The listing builds one solid part. Answer for the finished solid, in the listing's coordinates (mm). Face numbers are marked on the shaded views. A direction names the side the tool comes from. Coordinates: 2 decimals unless noted, no trailing zeros. Write each loop counter-clockwise with the first axis right and the second up, starting at its lowest first coordinate (ties: lowest second). Pieces come first, ordered by that corner, then holes. Notation, with made-up numbers: M 85.5,75.5 L 134.5,75.5 A17 ccw 134.5,108.5 Z; hole C 16,14.25 d3. An arc over 180 degrees is marked long. Answer as CSV lines item,"result".
```python
from build123d import *

# Parameters (mm, degrees)
BOSS_EXTRUDE1_DEPTH      = 30
SKETCH2_W                = 50
SKETCH2_H                = 10
CUT_EXTRUDE1_DEPTH       = 25
SKETCH4_R                = 1.5
BOSS_EXTRUDE2_DEPTH      = 5
SKETCH6_W                = 5.331604391
SKETCH6_H                = 3
SKETCH6_W_2              = 6.668395609
SKETCH6_W_3              = 12
SKETCH6_W_4              = 1.5
SKETCH6_H_2              = 4.5
CUT_EXTRUDE15_DEPTH      = 15
SKETCH7_W                = 30.5
SKETCH7_H                = 3
CUT_EXTRUDE16_DEPTH      = 13
CUT_EXTRUDE16_DEPTH_BACK = 3
SKETCH8_W                = 35
SKETCH8_H                = 39
CUT_EXTRUDE17_DEPTH      = 10
SKETCH3_W                = 35
SKETCH3_H                = 10
CUT_EXTRUDE18_DEPTH      = 40
SKETCH9_R                = 11.05
CUT_EXTRUDE19_DEPTH      = 8
FILLET5_R                = 5
FILLET6_R                = 5
FILLET7_R                = 5
FILLET8_R                = 5
FILLET9_R                = 5
FILLET10_R               = 5
SKETCH10_W               = 9
SKETCH10_H               = 10.2
CUT_EXTRUDE20_DEPTH      = 51
SKETCH11_R               = 1.5
BOSS_EXTRUDE3_DEPTH      = 5
SKETCH13_W               = 7.135367733
SKETCH13_H               = 3
SKETCH13_W_2             = 4.864632267
SKETCH13_W_3             = 12
CUT_EXTRUDE22_DEPTH      = 15
SKETCH14_W               = 21
SKETCH14_H               = 5
BOSS_EXTRUDE4_DEPTH      = 7.5
SKETCH15_W               = 21
SKETCH15_H               = 5
BOSS_EXTRUDE5_DEPTH      = 7.5
CUT_EXTRUDE23_DEPTH      = 3.5
SKETCH17_R               = 1.425
CUT_EXTRUDE24_DEPTH      = 2.5
SKETCH19_W               = 7.5
SKETCH19_H               = 10
BOSS_EXTRUDE7_DEPTH      = 9.5
FILLET14_R               = 5
FILLET18_R               = 5
FILLET19_R               = 5
FILLET20_R               = 5
FILLET21_R               = 5
FILLET22_R               = 5
FILLET23_R               = 5
FILLET24_R               = 5
SKETCH20_R               = 1.375
CUT_EXTRUDE25_DEPTH      = 10
SKETCH21_R               = 5.5
CUT_EXTRUDE26_DEPTH      = 10
CUT_EXTRUDE27_DEPTH      = 14
CUT_EXTRUDE27_DEPTH_BACK = 3


with BuildPart() as part:
    # Sketch1 → Boss-Extrude1 (new body)
    with BuildSketch(Plane.XY):
        Polygon((19.499094274, 17.872269618), (0.583421555, 17.872269618), (-16.737086521, 7.872269618), (-16.737086521, -47.127730382), (33.262913479, -47.127730382), (33.262913479, 7.872269618), align=None)
    extrude(amount=BOSS_EXTRUDE1_DEPTH)

    # Sketch2 → Cut-Extrude1 (cut)
    with BuildSketch(Plane(origin=(0, 17.872269618, 0), x_dir=(1, 0, 0), z_dir=(0, 1, 0))):
        with Locations((8.262913479, -15)):
            Rectangle(SKETCH2_W, SKETCH2_H)
    extrude(amount=-CUT_EXTRUDE1_DEPTH, mode=Mode.SUBTRACT)

    # Sketch4 → Boss-Extrude2 (add)
    with BuildSketch(Plane(origin=(-7.593064367, 13.151573269, 0), x_dir=(0, 0, 1), z_dir=(-0.5, 0.866025404, 0))):
        with Locations((10, 3.241392696)):
            Circle(SKETCH4_R)
        with Locations((20, 3.241392696)):
            Circle(SKETCH4_R)
    extrude(amount=-BOSS_EXTRUDE2_DEPTH)

    # Sketch6 → Cut-Extrude15 (cut)
    with BuildSketch(Plane(origin=(0, 17.872269618, 0), x_dir=(1, 0, 0), z_dir=(0, 1, 0))):
        with Locations((3.249223751, -7)):
            Rectangle(SKETCH6_W, SKETCH6_H)
        with Locations((-2.75077625, -7)):
            Rectangle(SKETCH6_W_2, SKETCH6_H)
        with Locations((-0.084974054, -23)):
            Rectangle(SKETCH6_W_3, SKETCH6_H)
        Polygon((-6.084974054, -24.5), (-6.084974054, -21.5), (-6.084974054, -20), (-7.584974054, -20), (-7.584974054, -24.5), align=None)
        with Locations((-6.834974054, -7.75)):
            Rectangle(SKETCH6_W_4, SKETCH6_H_2)
    extrude(amount=-CUT_EXTRUDE15_DEPTH, mode=Mode.SUBTRACT)

    # Sketch7 → Cut-Extrude16 (cut, two sides)
    with BuildSketch(Plane.XY.offset(10)) as cut_extrude16_sk:
        with Locations((9.165025946, 4.372269618)):
            Rectangle(SKETCH7_W, SKETCH7_H)
    extrude(amount=CUT_EXTRUDE16_DEPTH, mode=Mode.SUBTRACT)
    extrude(cut_extrude16_sk.sketch, amount=-CUT_EXTRUDE16_DEPTH_BACK, mode=Mode.SUBTRACT)

    # Sketch8 → Cut-Extrude17 (cut)
    with BuildSketch(Plane.XY.offset(30)):
        with Locations((8.262913479, -27.627730382)):
            Rectangle(SKETCH8_W, SKETCH8_H)
    extrude(amount=-CUT_EXTRUDE17_DEPTH, mode=Mode.SUBTRACT)

    # Sketch3 → Cut-Extrude18 (cut)
    with BuildSketch(Plane.XZ.offset(47.127730382)):
        with Locations((8.262913479, 15)):
            Rectangle(SKETCH3_W, SKETCH3_H)
    extrude(amount=-CUT_EXTRUDE18_DEPTH, mode=Mode.SUBTRACT)

    # Sketch9 → Cut-Extrude19 (cut)
    with BuildSketch(Plane.XY.offset(10)):
        with Locations((6.889118081, -18.127730382)):
            Circle(SKETCH9_R)
    extrude(amount=-CUT_EXTRUDE19_DEPTH, mode=Mode.SUBTRACT)

    # Fillet5
    fillet5_edges = [part.edges().sort_by_distance(p)[0] for p in [
        (-16.737086521, 7.872269618, 5),
    ]]
    fillet(fillet5_edges, radius=FILLET5_R)

    # Fillet6
    fillet6_edges = [part.edges().sort_by_distance(p)[0] for p in [
        (-16.737086521, 7.872269618, 25),
    ]]
    fillet(fillet6_edges, radius=FILLET6_R)

    # Fillet7
    fillet7_edges = [part.edges().sort_by_distance(p)[0] for p in [
        (0.583421555, 17.872269618, 2.75),
    ]]
    fillet(fillet7_edges, radius=FILLET7_R)

    # Fillet8
    fillet8_edges = [part.edges().sort_by_distance(p)[0] for p in [
        (0.583421555, 17.872269618, 9.25),
    ]]
    fillet(fillet8_edges, radius=FILLET8_R)

    # Fillet9
    fillet9_edges = [part.edges().sort_by_distance(p)[0] for p in [
        (0.583421555, 17.872269618, 20.75),
    ]]
    fillet(fillet9_edges, radius=FILLET9_R)

    # Fillet10
    fillet10_edges = [part.edges().sort_by_distance(p)[0] for p in [
        (0.583421555, 17.872269618, 27.25),
    ]]
    fillet(fillet10_edges, radius=FILLET10_R)

    # Sketch10 → Cut-Extrude20 (cut, through all)
    with BuildSketch(Plane(origin=(33.262913479, 0, 0), x_dir=(0, 0, -1), z_dir=(1, 0, 0))):
        with Locations((-25.5, -42.027730382)):
            Rectangle(SKETCH10_W, SKETCH10_H)
    extrude(amount=-CUT_EXTRUDE20_DEPTH, mode=Mode.SUBTRACT)

    # Sketch11 → Boss-Extrude3 (add)
    with BuildSketch(Plane(origin=(15.235540625, 20.969922665, 0), x_dir=(0, 0, -1), z_dir=(0.587785252, 0.809016994, 0))):
        with Locations((-20, -9.783058304)):
            Circle(SKETCH11_R)
        with Locations((-10, -9.783058304)):
            Circle(SKETCH11_R)
    extrude(amount=-BOSS_EXTRUDE3_DEPTH)

    # Sketch13 → Cut-Extrude22 (cut)
    with BuildSketch(Plane(origin=(0, 17.872269618, 0), x_dir=(1, 0, 0), z_dir=(0, 1, 0))):
        with Locations((15.931410407, -23)):
            Rectangle(SKETCH13_W, SKETCH13_H)
        with Locations((21.931410408, -23)):
            Rectangle(SKETCH13_W_2, SKETCH13_H)
        Polygon((24.363726541, -21.5), (24.363726541, -24.5), (25.363726541, -24.5), (25.363726541, -14.929315396), (24.363726541, -14.929315396), align=None)
        Polygon((24.363726541, -5.5), (24.363726541, -8.5), (24.363726541, -11.278829463), (25.363726541, -11.278829463), (25.363726541, -5.5), align=None)
        with Locations((18.363726541, -7)):
            Rectangle(SKETCH13_W_3, SKETCH13_H)
    extrude(amount=-CUT_EXTRUDE22_DEPTH, mode=Mode.SUBTRACT)

    # Sketch14 → Boss-Extrude4 (add)
    with BuildSketch(Plane.ZY.offset(16.737086521)):
        with Locations((10.5, -44.627730382)):
            Rectangle(SKETCH14_W, SKETCH14_H)
    extrude(amount=BOSS_EXTRUDE4_DEPTH)

    # Sketch15 → Boss-Extrude5 (add)
    with BuildSketch(Plane(origin=(33.262913479, 0, 0), x_dir=(0, 0, -1), z_dir=(1, 0, 0))):
        with Locations((-10.5, -44.627730382)):
            Rectangle(SKETCH15_W, SKETCH15_H)
    extrude(amount=BOSS_EXTRUDE5_DEPTH)

    # Sketch16 → Cut-Extrude23 (cut)
    with BuildSketch(Plane(origin=(0, -42.127730382, 0), x_dir=(1, 0, 0), z_dir=(0, 1, 0))):
        Polygon((37.012913479, -11.651368439), (34.112913479, -13.325684219), (34.112913479, -16.674315781), (37.012913479, -18.348631561), (39.912913479, -16.674315781), (39.912913479, -13.325684219), align=None)
        Polygon((37.012913479, -1.651368439), (34.112913479, -3.325684219), (34.112913479, -6.674315781), (37.012913479, -8.348631561), (39.912913479, -6.674315781), (39.912913479, -3.325684219), align=None)
    extrude(amount=-CUT_EXTRUDE23_DEPTH, mode=Mode.SUBTRACT)

    # Sketch17 → Cut-Extrude24 (cut, through all)
    with BuildSketch(Plane(origin=(0, -45.627730382, 0), x_dir=(1, 0, 0), z_dir=(0, 1, 0))):
        with Locations((37.012913479, -15)):
            Circle(SKETCH17_R)
        with Locations((37.012913479, -5)):
            Circle(SKETCH17_R)
    extrude(amount=-CUT_EXTRUDE24_DEPTH, mode=Mode.SUBTRACT)

    # Sketch19 → Boss-Extrude7 (add)
    with BuildSketch(Plane(origin=(0, -7.127730382, 0), x_dir=(1, 0, 0), z_dir=(0, 1, 0))):
        with Locations((-12.987086521, -15)):
            Rectangle(SKETCH19_W, SKETCH19_H)
        with Locations((29.512913479, -15)):
            Rectangle(SKETCH19_W, SKETCH19_H)
    extrude(amount=BOSS_EXTRUDE7_DEPTH)

    # Fillet14
    fillet14_edges = [part.edges().sort_by_distance(p)[0] for p in [
        (-9.237086521, 2.372269618, 15),
    ]]
    fillet(fillet14_edges, radius=FILLET14_R)

    # Fillet18
    fillet18_edges = [part.edges().sort_by_distance(p)[0] for p in [
        (25.762913479, 2.372269618, 15),
    ]]
    fillet(fillet18_edges, radius=FILLET18_R)

    # Fillet19
    fillet19_edges = [part.edges().sort_by_distance(p)[0] for p in [
        (33.262913479, 7.872269618, 5),
    ]]
    fillet(fillet19_edges, radius=FILLET19_R)

    # Fillet20
    fillet20_edges = [part.edges().sort_by_distance(p)[0] for p in [
        (33.262913479, 7.872269618, 25),
    ]]
    fillet(fillet20_edges, radius=FILLET20_R)

    # Fillet21
    fillet21_edges = [part.edges().sort_by_distance(p)[0] for p in [
        (19.499094274, 17.872269618, 2.75),
    ]]
    fillet(fillet21_edges, radius=FILLET21_R)

    # Fillet22
    fillet22_edges = [part.edges().sort_by_distance(p)[0] for p in [
        (19.499094274, 17.872269618, 9.25),
    ]]
    fillet(fillet22_edges, radius=FILLET22_R)

    # Fillet23
    fillet23_edges = [part.edges().sort_by_distance(p)[0] for p in [
        (19.499094274, 17.872269618, 27.25),
    ]]
    fillet(fillet23_edges, radius=FILLET23_R)

    # Fillet24
    fillet24_edges = [part.edges().sort_by_distance(p)[0] for p in [
        (19.499094274, 17.872269618, 20.75),
    ]]
    fillet(fillet24_edges, radius=FILLET24_R)

    # Sketch20 → Cut-Extrude25 (cut)
    with BuildSketch(Plane(origin=(0, -42.127730382, 0), x_dir=(1, 0, 0), z_dir=(0, 1, 0))):
        with Locations((-20.537086521, -11)):
            Circle(SKETCH20_R)
    extrude(amount=-CUT_EXTRUDE25_DEPTH, mode=Mode.SUBTRACT)

    # Sketch21 → Cut-Extrude26 (cut)
    with BuildSketch(Plane.XY.offset(2)):
        with Locations((6.889118081, -18.127730382)):
            Circle(SKETCH21_R)
    extrude(amount=-CUT_EXTRUDE26_DEPTH, mode=Mode.SUBTRACT)

    # Sketch22 → Cut-Extrude27 (cut, two sides)
    with BuildSketch(Plane.XY.offset(10)) as cut_extrude27_sk:
        Polygon((-2.084974054, 5.872269618), (-6.084974054, 12.872269618), (-6.084974054, 5.872269618), align=None)
        Polygon((24.363726541, 13.372269618), (18.863726541, 5.872269618), (24.363726541, 5.872269618), align=None)
    extrude(amount=CUT_EXTRUDE27_DEPTH, mode=Mode.SUBTRACT)
    extrude(cut_extrude27_sk.sketch, amount=-CUT_EXTRUDE27_DEPTH_BACK, mode=Mode.SUBTRACT)


solid = part.part
```
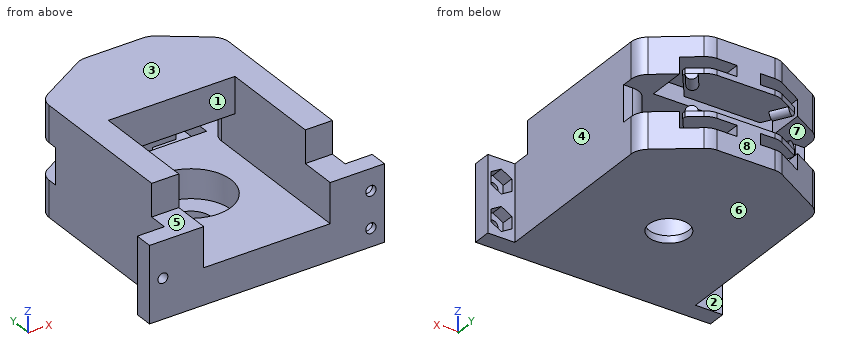
Q1. Straight lines are drawn through the part: line 1 (X direction, y = -44.65, z = 11); line 2 (X direction, y = -29.5, z = 19.25); line 3 (X direction, y = 13, z = 22.25). For each, find the intervals that lie inside material, in ascending order.
Output:
line 1,"-24.24 to -21.91, -19.16 to -9.24, 25.76 to 40.76"
line 2,"-16.74 to -9.24, 25.76 to 33.26"
line 3,"-7.86 to -7.58, 5.92 to 12.36, 25.36 to 26.21"
Q2. Flat-ended cylindrical pins translate along their axes: pin 1 Ø3.5 at (x, y) = (18, 10) entering from -Z; pin 2 Ø10 at (y, z) = (-38.5, 27) entering from -X; pin 3 Ø4 at (x, y) = (22.5, -35) entering from +Z; pin 4 Ø1.5 at (y, z) = (10.5, 22.5) entering from -X. Find the tip coordinate at first contact, or state that the pin passes through.
Output:
pin 1,"z = 0"
pin 2,"x = -16.74"
pin 3,"z = 10"
pin 4,"x = -13.48"
Q3. Find section B-B (z = 25.75). Give the vertices of the cut face in (x, y).
Output:
outline,"M -16.74,-36.93 L -9.24,-36.93 L -9.24,-8.13 L 25.76,-8.13 L 25.76,-36.93 L 33.26,-36.93 L 33.26,5.32 A5 ccw 31.2,9.37 L 20.81,16.92 A5 ccw 17.87,17.87 L 1.92,17.87 A5 ccw -0.58,17.2 L -14.24,9.32 A5 ccw -16.74,4.99 Z"
Q4. The mould has two halves that part along Z. Classify the marked faces 6, 7 and 8: pulls with the +Z half, pulls with the -Z half, needs draft (parallel to the pull), parting line crosses it, or undercut.
Output:
face 6,"pulls with the -Z half"
face 7,"undercut"
face 8,"needs draft"
Q5. For the marked faces 1, 2, 3, 4 and 5, determine the directions among +Z, -Z, +X, -X, +Y, -Y from which every point of the face is accessible in a straight line to the end or side of a thin tool.
Output:
face 1,"+Z, -Y"
face 2,"+Z, -Z, -X, +Y"
face 3,"+Z, +X, -X, +Y, -Y"
face 4,"+Z, -Z, +X, +Y"
face 5,"+Z, +X, -X, -Y"
Q6. Find section C-C (y = -38). Give the vertices of the cut face in (x, z), and give its area (3 significant figures).
Output:
outline,"M -16.74,0 L 33.26,0 L 33.26,21 L 25.76,21 L 25.76,10 L -9.24,10 L -9.24,21 L -16.74,21 Z"
area,"665 mm2"
Q7. Find section A-A (z = 15). Give the vertices of the cut face in (x, y).
Output:
outline,"M -24.24,-47.13 L -9.24,-47.13 L -9.24,-2.63 A5 ccw -14.24,2.37 L -16.74,2.37 L -16.74,-42.13 L -24.24,-42.13 Z; M 25.76,-47.13 L 35.59,-47.13 L 35.59,-45.63 L 34.11,-45.63 L 34.11,-42.13 L 33.26,-42.13 L 33.26,2.37 L 30.76,2.37 A5 ccw 25.76,-2.63 Z; M 38.44,-47.13 L 40.76,-47.13 L 40.76,-42.13 L 39.91,-42.13 L 39.91,-45.63 L 38.44,-45.63 Z"
Q8. Find section D-D (x = 9.5). Give the vertices of the cut face in (y, z), and give its area (3 significant figures).
Output:
outline,"M -47.13,0 L -22.97,0 L -22.97,2 L -28.86,2 L -28.86,10 L -47.13,10 Z; M -13.29,0 L 17.87,0 L 17.87,10 L 5.87,10 L 5.87,7 L 2.87,7 L 2.87,10 L -7.39,10 L -7.39,2 L -13.29,2 Z; M -8.13,20 L 2.87,20 L 2.87,23 L 5.87,23 L 5.87,20 L 17.87,20 L 17.87,30 L -8.13,30 Z"
area,"701 mm2"
